from build123d import *

# Parameters (mm, degrees)
SKETCH_1_R          = 32.5
EXTRUDE_1_DEPTH     = 26
SKETCH_3_R          = 26
CUT_EXTRUDE_1_DEPTH = 53.80624963
FILLET_1_R          = 2


with BuildPart() as part:
    # 草图1 → 凸台-拉伸1 (new body)
    with BuildSketch(Plane(origin=(0, 0, 0), x_dir=(1, 0, 0), z_dir=(0, 1, 0))):
        with Locations(Location((0, 0, 0), (0, 0, 90))):
            Circle(SKETCH_1_R)
    extrude(amount=EXTRUDE_1_DEPTH)

    # 草图3 → 切除-拉伸1 (cut, through all)
    with BuildSketch(Plane(origin=(0, 26, 0), x_dir=(1, 0, 0), z_dir=(0, 1, 0))):
        with Locations(Location((0, 0, 0), (0, 0, 270))):
            Circle(SKETCH_3_R)
    extrude(amount=-CUT_EXTRUDE_1_DEPTH, mode=Mode.SUBTRACT)

    # 圆角1
    fillet_1_edges = [part.edges().sort_by_distance(p)[0] for p in [
        (0, 0, 32.5),
        (0, 26, 32.5),
    ]]
    fillet(fillet_1_edges, radius=FILLET_1_R)


solid = part.part
The model under review builds one solid part; all positions refer to its coordinate system, in mm. Coordinates: 2 decimals unless noted, no trailing zeros. Write each loop counter-clockwise with the first axis right and the second up, starting at its lowest first coordinate (ties: lowest second). Pieces come first, ordered by that corner, then holes. Notation, with made-up numbers: (74.5, 36) - (96.5, 36) arc R24 cw to (96.5, 73) - close; hole circle Ø11 at (-31, 3). An arc over 180 degrees is marked (long way). Answer as a JSON object with one key per item and string values. Group by question number.
1. Add section B-B (y = 6). Give the boundary of the cut face in (x, z), plus the area to 3 significant figures.
2. To check wall thickness, follow probe 1 along X at (y, z) = (4.75, -0.5); probe 2 along Z at (x, y) = (3.5, 24.5). State the ranges of each line that lie inside material, in increasing order.
3. Add section A-A (z = 0). Give the boundary of the cut face in (x, y), plus the area to 3 significant figures.
4. Mouldability with a two-part tool opening along Z and no side actions: class faces 1 (the face through (-13.7, 26, -22.5)), 2 (the face through (-9.76, 12.85, -31)), 3 (the face through (-15.821, 13.182, -20.633)) as pulls with the +Z half, pulls with the -Z half, needs draft (parallel to the pull), parting line crosses it, or undercut.
5. Clearance check with flat-ended pins moving along their axes: pin 1 Ø1.5 at (y, z) = (14.5, -4) entering from +X; pin 2 Ø1.5 at (y, z) = (18.5, 25) entering from -X; pin 3 Ø1 at (y, z) = (13, 20) entering from -X. State where each tip first meets the part, or that it passes through.
Findings:
{
 "1": {"outline": "circle Ø65 at (0, 0); hole circle Ø52 at (0, 0)", "area": "1,190 mm²"},
 "2": {"probe 1": "-32.5 to -26, 26 to 32.5", "probe 2": "-32.25 to -25.76, 25.76 to 32.25"},
 "3": {"outline": "(-32.5, 2) arc R2 ccw to (-30.5, 0) - (-26, 0) - (-26, 26) - (-30.5, 26) arc R2 ccw to (-32.5, 24) - close; (26, 0) - (30.5, 0) arc R2 ccw to (32.5, 2) - (32.5, 24) arc R2 ccw to (30.5, 26) - (26, 26) - close", "area": "335 mm²"},
 "4": {"face 1": "needs draft", "face 2": "parting line crosses it", "face 3": "undercut"},
 "5": {"pin 1": "x = 32.34", "pin 2": "x = -21.64", "pin 3": "x = -26"}
}
